```python
from build123d import *

# Parameters (mm, degrees)
SKETCH1_R           = 1
SKETCH1_R_2         = 1.5
BOSS_EXTRUDE1_DEPTH = 2
CUT_EXTRUDE1_DEPTH  = 14


with BuildPart() as part:
    # Sketch1 → Boss-Extrude1 (new body)
    with BuildSketch(Plane.XY):
        with BuildLine():
            Line((-0.5, 22.5), (0.5, 22.5))
            ThreePointArc((0.5, 22.5), (2.621320344, 21.621320344), (3.5, 19.5))
            Line((3.5, 19.5), (3.5, -19.5))
            ThreePointArc((3.5, -19.5), (2.621320344, -21.621320344), (0.5, -22.5))
            Line((0.5, -22.5), (-0.5, -22.5))
            ThreePointArc((-0.5, -22.5), (-2.621320344, -21.621320344), (-3.5, -19.5))
            Line((-3.5, -19.5), (-3.5, 19.5))
            ThreePointArc((-3.5, 19.5), (-2.621320344, 21.621320344), (-0.5, 22.5))
        make_face()
        with Locations((0, 19)):
            Circle(SKETCH1_R, mode=Mode.SUBTRACT)
        with Locations((0, -19)):
            Circle(SKETCH1_R_2, mode=Mode.SUBTRACT)
    extrude(amount=BOSS_EXTRUDE1_DEPTH)

    # Sketch2 → Cut-Extrude1 (cut)
    with BuildSketch(Plane.XY.offset(2)):
        with BuildLine():
            Line((-3.5, 14.530463873), (-3.5, -15.069881222))
            add(Edge.make_bspline(
                [(-3.5, 14.530463873), (-0.195046467, -0.263066887), (-3.5, -15.069881222)],
                knots=[0, 0, 0, 1, 1, 1], degree=2))
        make_face()
        with BuildLine():
            add(Edge.make_bspline(
                [(3.5, 14.530463873), (0.195046467, -0.263066887), (3.5, -15.069881222)],
                knots=[0, 0, 0, 1, 1, 1], degree=2))
            Line((3.5, -15.069881222), (3.5, 14.530463873))
        make_face()
    extrude(amount=-CUT_EXTRUDE1_DEPTH, mode=Mode.SUBTRACT)


solid = part.part
```
Could you check a few things on this model? Use its own coordinates, in mm. Coordinates: 2 decimals unless noted, no trailing zeros. Write each loop counter-clockwise with the first axis right and the second up, starting at its lowest first coordinate (ties: lowest second). Pieces come first, ordered by that corner, then holes. Notation, with made-up numbers: (-15.75, -30.75) -> (19.25, -30.75) arc R17 ccw to (19.25, -22.75) -> close; hole circle Ø1 at (70, 8). An arc over 180 degrees is marked (long way). One line per question, with ' | ' between items. Start each with the question number.
1. Thinking about a two-plate mould opening in Y: for faces 1 (the face through (2.6, 21.64, 0.99)), 2 (the face through (-3.5, 17, 1)), 3 (the face through (0, 18, 1)), 4 (the face through (2.64, -21.6, 0.99)), which applies, pulls with the +Y half, pulls with the -Y half, needs draft (parallel to the pull), parting line crosses it, or undercut?
2. Please list where these lines run through material, in increasing order: line 1 along Y through (x, z) = (0, 0.55); line 2 along Y through (x, z) = (-0.5, 0.6); line 3 along X through (y, z) = (7, 1.35).
3. If we section it at D-D (z = 0.45): Count the separate pieces of the cut face and the enclosed holes in it, and give its area (3 significant figures).
4. If we section it at A-A (y = -19): Please give me the cut outline in (x, z).
5. If we section it at C-C (y = 19): Please give me the cut outline in (x, z).
6. If we section it at B-B (x = 0): Please give me the cut outline in (y, z).
Return value:
1) face 1: pulls with the +Y half | face 2: needs draft | face 3: undercut | face 4: pulls with the -Y half
2) line 1: y = -22.5 to -20.5, -17.5 to 18, 20 to 22.5 | line 2: y = -22.5 to -20.41, -17.59 to 18.13, 19.87 to 22.5 | line 3: x = -2.25 to 2.25
3) separate pieces: 1 | enclosed holes: 2 | area: 232 mm²
4) outline: (-3.5, 0) -> (-1.5, 0) -> (-1.5, 2) -> (-3.5, 2) -> close; (1.5, 0) -> (3.5, 0) -> (3.5, 2) -> (1.5, 2) -> close
5) outline: (-3.5, 0) -> (-1, 0) -> (-1, 2) -> (-3.5, 2) -> close; (1, 0) -> (3.5, 0) -> (3.5, 2) -> (1, 2) -> close
6) outline: (-22.5, 0) -> (-20.5, 0) -> (-20.5, 2) -> (-22.5, 2) -> close; (-17.5, 0) -> (18, 0) -> (18, 2) -> (-17.5, 2) -> close; (20, 0) -> (22.5, 0) -> (22.5, 2) -> (20, 2) -> close
